The model under review builds one solid part; all positions refer to its coordinate system, in mm. Face numbers are marked on the shaded views. A direction names the side the tool comes from. Coordinates: 2 decimals unless noted, no trailing zeros. Order: outer loops, then holes, each group sorted by start corner. A loop starts at its lowest first (then second) coordinate and runs counter-clockwise, first axis right, second up. Notation, with made-up numbers: (33.5, 21.25) - (48.5, 21.25) arc R26 cw to (48.5, 35.25) - close; hole circle Ø2 at (65.25, 45). An arc over 180 degrees is marked (long way). Answer in a Markdown table with one row per item.
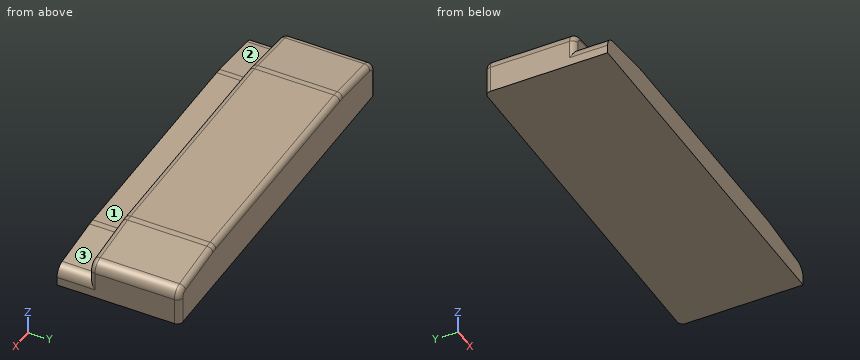
```python
from build123d import *

# Parameters (mm, degrees)
BOSS_EXTRUDE1_DEPTH = 168.275
CUT_EXTRUDE1_DEPTH  = 44.45
FILLET1_R           = 15.24
FILLET2_R           = 76.2
FILLET3_R           = 7.62
FILLET4_R           = 7.62


with BuildPart() as part:
    # Sketch7 → Boss-Extrude1 (new body)
    with BuildSketch(Plane(origin=(0, 0, 0), x_dir=(1, 0, 0), z_dir=(0, 1, 0))):
        Polygon((0, 0), (508, 0), (508, -50.8), (419.1, -60.325), (88.9, -60.325), (0, -50.8), align=None)
    extrude(amount=BOSS_EXTRUDE1_DEPTH)

    # Sketch10 → Cut-Extrude1 (cut)
    with BuildSketch(Plane.XZ):
        Polygon((0, 50.8), (0, 25.4), (88.9, 34.925), (419.1, 34.925), (508, 25.4), (508, 50.8), (419.1, 60.325), (88.9, 60.325), align=None)
    extrude(amount=-CUT_EXTRUDE1_DEPTH, mode=Mode.SUBTRACT)

    # Fillet1
    fillet1_edges = [part.edges().sort_by_distance(p)[0] for p in [
        (508, 106.3625, 50.8),
        (0, 106.3625, 50.8),
        (508, 22.225, 25.4),
        (0, 22.225, 25.4),
    ]]
    fillet(fillet1_edges, radius=FILLET1_R)

    # Fillet2
    fillet2_edges = [part.edges().sort_by_distance(p)[0] for p in [
        (419.1, 106.3625, 60.325),
        (88.9, 106.3625, 60.325),
        (419.1, 22.225, 34.925),
        (88.9, 22.225, 34.925),
    ]]
    fillet(fillet2_edges, radius=FILLET2_R)

    # Fillet3
    fillet3_edges = [part.edges().sort_by_distance(p)[0] for p in [
        (508, 168.275, 18.552816133),
        (0, 168.275, 18.552816133),
        (49.234552732, 168.275, 56.07513065),
        (3.904199904, 168.275, 47.291761863),
        (504.095800096, 168.275, 47.291761863),
        (458.765447268, 168.275, 56.07513065),
        (254, 168.275, 60.325),
        (88.905795265, 168.275, 60.216512154),
        (419.094204735, 168.275, 60.216512154),
    ]]
    fillet(fillet3_edges, radius=FILLET3_R)

    # Fillet4
    fillet4_edges = [part.edges().sort_by_distance(p)[0] for p in [
        (508, 44.45, 18.552816133),
        (0, 44.45, 18.552816133),
        (458.765447268, 44.45, 56.07513065),
        (3.904199904, 44.45, 47.291761863),
        (504.095800096, 44.45, 47.291761863),
        (254, 44.45, 60.325),
        (49.234552732, 44.45, 56.07513065),
        (88.905795265, 44.45, 60.216512154),
        (419.094204735, 44.45, 60.216512154),
    ]]
    fillet(fillet4_edges, radius=FILLET4_R)


solid = part.part
```
Item 1: To check wall thickness, follow line 1 (Z direction, x = 302, y = 18) (3 decimals); line 2 (X direction, y = 138, z = 38.5); line 3 (Y direction, x = 461, z = 49). State the ranges of each line that lie inside material, in increasing order. Write a range as from..to.
Check values:
| item | result |
|---|---|
| line 1 | 0..34.925 |
| line 2 | 0.06..507.94 |
| line 3 | 44.49..168.23 |
Item 2: Tool access review of the marked faces 1, 2 and 3: name each direction out of +Z, -Z, +X, -X, +Y, -Y from which nothing blocks a thin tool from reaching the whole face with its end or side.
Check values:
| item | result |
|---|---|
| face 1 | +Z, +X, -X, -Y |
| face 2 | +Z, -X, -Y |
| face 3 | +Z, +X, -Y |
Item 3: We need section B-B, the plane x = 398. Write out the cut boundary in (y, z) (3 decimals), then the cut area to 3 significant figures.
Check values:
| item | result |
|---|---|
| outline | (0, 0) - (168.275, 0) - (168.275, 52.705) arc R7.62 ccw to (160.655, 60.325) - (52.07, 60.325) arc R7.62 ccw to (44.45, 52.705) - (44.45, 34.925) - (0, 34.925) - close |
| area | 9,000 mm^2 |
Item 4: Clearance check with flat-ended pins moving along their axes: pin 1 Ø8 at (y, z) = (21.5, 16.5) entering from -X; pin 2 Ø1.5 at (y, z) = (49, 51) entering from -X; pin 3 Ø22 at (x, y) = (200.5, 18.5) entering from +Z (3 decimals). State where each tip first meets the part, or that it passes through.
Check values:
| item | result |
|---|---|
| pin 1 | x = 0.02 |
| pin 2 | x = 8.74 |
| pin 3 | z = 34.925 |
Item 5: We need section A-A, the plane y = 143. Write out the cut boundary in (x, z) (1 decimal).
Check values:
| item | result |
|---|---|
| outline | (0, 0) - (508, 0) - (508, 37.1) arc R15.2 ccw to (494.4, 52.3) - (423.1, 59.9) arc R76.2 ccw to (415, 60.3) - (93, 60.3) arc R76.2 ccw to (84.9, 59.9) - (13.6, 52.3) arc R15.2 ccw to (0, 37.1) - close |
